Part print with two shaded views. Sizes in mm from the minimum x, y, z corner. A direction names the side the tool comes from. Round coordinates to 2 decimals unless told otherwise and drop trailing zeros. Loops run counter-clockwise (first coordinate to the right, second up) from the corner with the lowest first, then second, coordinate; pieces in that order, holes last.
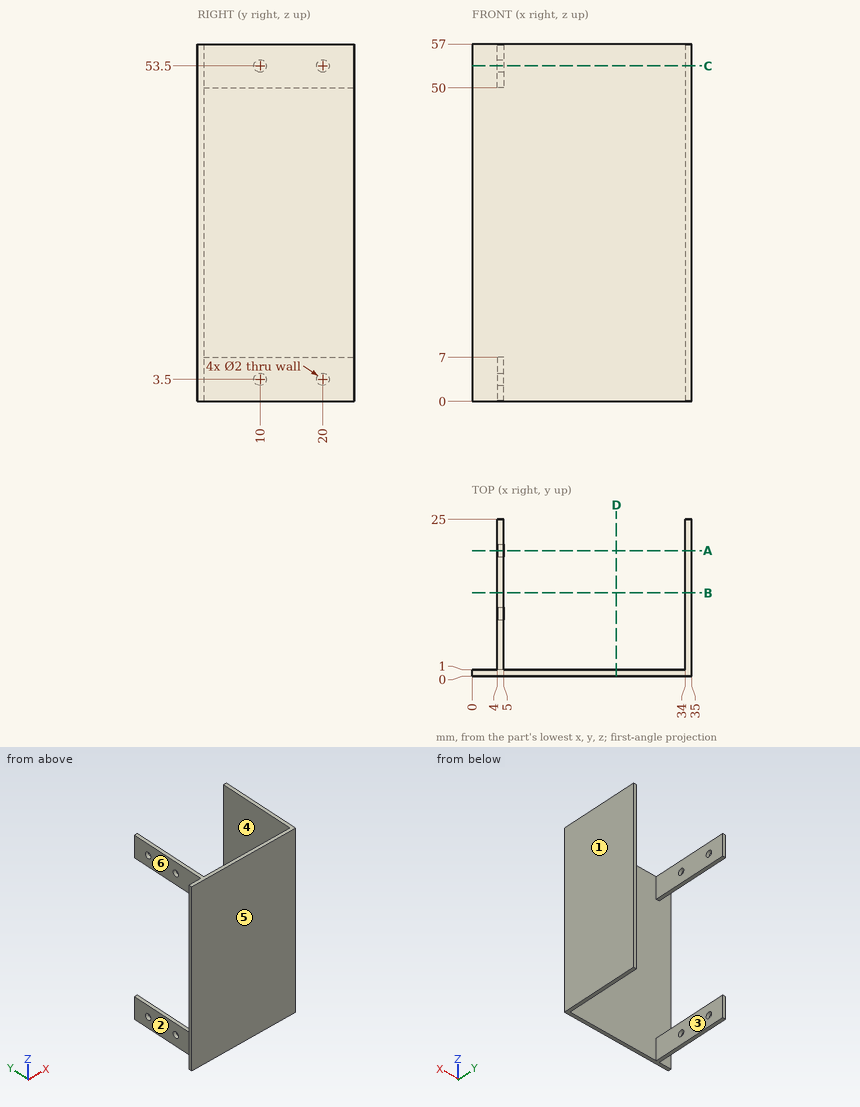
Item 1: Mould opens along X. For the marked faces 1, 2 and 3 say: released by +X, released by -X, zero draft, split by the parting line, or undercut.
Verdict:
face 1: released by +X
face 2: released by -X
face 3: undercut
Item 2: Wall check: L1, parallel to Z at x = 4.75, y = 10; L2, parallel to Y at x = 4.4, z = 3.5; L3, parallel to X at y = 22.75, z = 54.5. Give the ranges that are in metal, low to high.
Verdict:
L1: z = 0 to 2.5, 4.5 to 7, 50 to 52.5, 54.5 to 57
L2: y = 0 to 9, 11 to 19, 21 to 25
L3: x = 4 to 5, 34 to 35
Item 3: Cut at C-C (z = 53.5). List the corners of the cut face in (x, y).
Verdict:
outline: (0, 0) - (35, 0) - (35, 25) - (34, 25) - (34, 1) - (5, 1) - (5, 9) - (4, 9) - (4, 1) - (0, 1) - close; (4, 11) - (5, 11) - (5, 19) - (4, 19) - close; (4, 21) - (5, 21) - (5, 25) - (4, 25) - close
Item 4: Cut at D-D (x = 23). List the corners of the cut face in (y, z), plus the area to 3 significant figures.
Verdict:
outline: (0, 0) - (1, 0) - (1, 57) - (0, 57) - close
area: 57.0 mm2
Item 5: Flat gauge pins, fed straight in: P1, Ø1.6, axis at y = 20, z = 3.5, coming from the -X side; P2, Ø12, axis at y = 10, z = 49.5, coming from the -X side; P3, Ø17, axis at x = 18.5, z = 37, coming from the +Y side. Where does each tip first touch, or does it go through?
Verdict:
P1: stops at x = 34
P2: stops at x = 4
P3: stops at y = 1
Item 6: Cut at B-B (y = 13.25). List the corners of the cut face in (x, z), plus the area to 3 significant figures.
Verdict:
outline: (4, 0) - (5, 0) - (5, 7) - (4, 7) - close; (4, 50) - (5, 50) - (5, 57) - (4, 57) - close; (34, 0) - (35, 0) - (35, 57) - (34, 57) - close
area: 71.0 mm2
Item 7: 3-axis set-ups, long thin cutter, end or side, ignore diameter. For the marked faces 4, 5 and 6: which of +Z, -Z, +X, -X, +Y, -Y reach the whole face in a straight line?
Verdict:
face 4: +Z, -Z, +Y
face 5: +Z, -Z, +X, -X, -Y
face 6: +Z, -Z, -X, +Y
Item 8: Cut at A-A (y = 20). List the corners of the cut face in (x, z), plus the area to 3 significant figures.
Verdict:
outline: (4, 0) - (5, 0) - (5, 2.5) - (4, 2.5) - close; (4, 4.5) - (5, 4.5) - (5, 7) - (4, 7) - close; (4, 50) - (5, 50) - (5, 52.5) - (4, 52.5) - close; (4, 54.5) - (5, 54.5) - (5, 57) - (4, 57) - close; (34, 0) - (35, 0) - (35, 57) - (34, 57) - close
area: 67.0 mm2
